The figure shows three views and two pictorial views of one solid part (mm, origin at its lowest corner). Answer the questions. Give positions to 0.01 mm unless a question says otherwise; leave off trailing zeros. Order: outer loops, then holes, each group sorted by start corner. A loop starts at its lowest first (then second) coordinate and runs counter-clockwise, first axis right, second up. Notation, with made-up numbers: (-32, -27) - (-27, -27) arc R32 cw to (-27, 5) - close; hole circle Ø9 at (-21.75, 74). An arc over 180 degrees is marked (long way). Answer as a JSON object with one key per item and string values. Group by question number.
Q1. A cutting plane is placed at C-C, the plane z = 1.1. Give the vertices of the cut face in (x, y).
Q2. A cutting plane is placed at D-D, the plane y = 48.5. Give the vertices of the cut face in (x, z).
Q3. Consider line 1 (X direction, y = 86, z = 1.85); line 2 (Y direction, x = 28, z = 2.4); line 3 (Y direction, x = 4, z = 1.15). Determine where each line is inside the solid, lowest interval first.
Q4. The mould has two halves that part along X. Classify the marked faces 1 and 2: released by +X, released by -X, zero draft, split by the parting line, or undercut.
Q5. Given pin 1 (8 mm diameter, centred on x = 12.5, y = 54.5, fed in from +Z); pin 2 (4 mm diameter, centred on x = 28, y = 86, fed in from -Z), each flat-ended and moving along its own axis, determine where each tip first touches the part or whether it passes through.
Q6. A cutting plane is placed at B-B, the plane y = 4. Give the vertices of the cut face in (x, z).
Q7. A cutting plane is placed at A-A, the plane x = 28. Give the vertices of the cut face in (y, z), and give its area (3 significant figures).
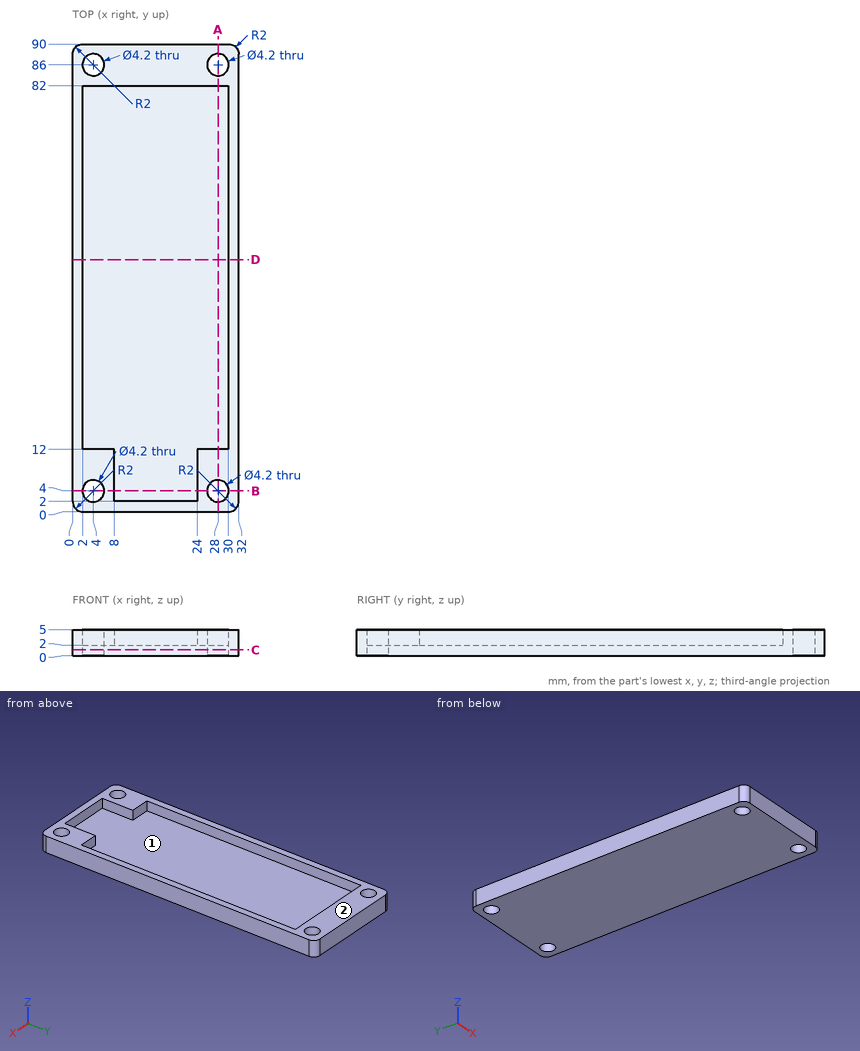
Reply:
{
 "1": {"outline": "(0, 2) arc R2 ccw to (2, 0) - (30, 0) arc R2 ccw to (32, 2) - (32, 88) arc R2 ccw to (30, 90) - (2, 90) arc R2 ccw to (0, 88) - close; hole circle Ø4.2 at (4, 4); hole circle Ø4.2 at (4, 86); hole circle Ø4.2 at (28, 4); hole circle Ø4.2 at (28, 86)"},
 "2": {"outline": "(0, 0) - (32, 0) - (32, 5) - (30, 5) - (30, 2) - (2, 2) - (2, 5) - (0, 5) - close"},
 "3": {"line 1": "x = 0 to 1.9, 6.1 to 25.9, 30.1 to 32", "line 2": "y = 0 to 1.9, 6.1 to 12, 82 to 83.9, 88.1 to 90", "line 3": "y = 0 to 1.9, 6.1 to 83.9, 88.1 to 90"},
 "4": {"face 1": "undercut", "face 2": "zero draft"},
 "5": {"pin 1": "stops at z = 2", "pin 2": "passes through"},
 "6": {"outline": "(0, 0) - (1.9, 0) - (1.9, 5) - (0, 5) - close; (6.1, 0) - (25.9, 0) - (25.9, 5) - (24, 5) - (24, 2) - (8, 2) - (8, 5) - (6.1, 5) - close; (30.1, 0) - (32, 0) - (32, 5) - (30.1, 5) - close"},
 "7": {"outline": "(0, 0) - (1.9, 0) - (1.9, 5) - (0, 5) - close; (6.1, 0) - (83.9, 0) - (83.9, 5) - (82, 5) - (82, 2) - (12, 2) - (12, 5) - (6.1, 5) - close; (88.1, 0) - (90, 0) - (90, 5) - (88.1, 5) - close", "area": "198 mm^2"}
}
